```python
from build123d import *

# Parameters (mm, degrees)
SKETCH1_R                    = 9.5
BOSS_EXTRUDE1_DEPTH          = 10
CHAMFER1_SIZE                = 0.75
CIRPATTERN1_COUNT            = 12
CHAMFER1_OF_CIRPATTERN1_SIZE = 0.75
SKETCH2_R                    = 7
SKETCH2_R_2                  = 4.5
CUT_EXTRUDE1_DEPTH           = 2
FILLET1_R                    = 1
FILLET1_OF_MIRROR1_R         = 1
CUT_EXTRUDE2_REACH           = 12


with BuildPart() as part:
    # Sketch1 → Boss-Extrude1 (new body)
    with BuildSketch(Plane.XY):
        Circle(SKETCH1_R)
        with BuildLine():
            ThreePointArc((-2.07, 9.271736623), (0, 9.5), (2.07, 9.271736623))
            ThreePointArc((2.07, 9.271736623), (1.625653209, 11.72726856), (0.57, 13.988391616))
            ThreePointArc((0.57, 13.988391616), (0, 14), (-0.57, 13.988391616))
            ThreePointArc((-0.57, 13.988391616), (-1.625653209, 11.72726856), (-2.07, 9.271736623))
        make_face()
    boss_extrude1 = extrude(amount=BOSS_EXTRUDE1_DEPTH)

    # Chamfer1
    chamfer1_edges = [part.edges().sort_by_distance(p)[0] for p in [
        (0, 14, 10),
        (0, 14, 0),
    ]]
    chamfer(chamfer1_edges, length=CHAMFER1_SIZE)

    # CirPattern1: Boss-Extrude1 ×12 about axis
    cirpattern1_axis = Axis((0, 0, 0), (0, 0, 1))
    for i in range(1, CIRPATTERN1_COUNT):
        add(boss_extrude1.rotate(cirpattern1_axis, i * 360 / CIRPATTERN1_COUNT))

    # Chamfer1 of CirPattern1
    chamfer1_of_cirpattern1_edges = [part.edges().sort_by_distance(p)[0] for p in [
        (-7, 12.124355653, 10),
        (-7, 12.124355653, 0),
        (-12.124355653, 7, 10),
        (-12.124355653, 7, 0),
        (-14, 0, 10),
        (-14, 0, 0),
        (-12.124355653, -7, 10),
        (-12.124355653, -7, 0),
        (-7, -12.124355653, 10),
        (-7, -12.124355653, 0),
        (0, -14, 10),
        (0, -14, 0),
        (7, -12.124355653, 10),
        (7, -12.124355653, 0),
        (12.124355653, -7, 10),
        (12.124355653, -7, 0),
        (14, 0, 10),
        (14, 0, 0),
        (12.124355653, 7, 10),
        (12.124355653, 7, 0),
        (7, 12.124355653, 10),
        (7, 12.124355653, 0),
    ]]
    chamfer(chamfer1_of_cirpattern1_edges, length=CHAMFER1_OF_CIRPATTERN1_SIZE)

    # Sketch2 → Cut-Extrude1 (cut)
    with BuildSketch(Plane.XY.offset(10)):
        Circle(SKETCH2_R)
        Circle(SKETCH2_R_2, mode=Mode.SUBTRACT)
    cut_extrude1 = extrude(amount=-CUT_EXTRUDE1_DEPTH, mode=Mode.SUBTRACT)

    # Fillet1
    fillet1_edges = [part.edges().sort_by_distance(p)[0] for p in [
        (-7, 0, 8),
        (-4.5, 0, 8),
    ]]
    fillet(fillet1_edges, radius=FILLET1_R)

    # Mirror1: Cut-Extrude1 across plane
    add(cut_extrude1.mirror(Plane.XY.offset(5)), mode=Mode.SUBTRACT)

    # Fillet1 of Mirror1
    fillet1_of_mirror1_edges = [part.edges().sort_by_distance(p)[0] for p in [
        (-7, 0, 2),
        (-4.5, 0, 2),
    ]]
    fillet(fillet1_of_mirror1_edges, radius=FILLET1_OF_MIRROR1_R)

    # Sketch3 → Cut-Extrude2 (cut, up to next)
    with BuildSketch(Plane.XY.offset(10), mode=Mode.PRIVATE) as cut_extrude2_sk1:
        with BuildLine():
            Line((1.2489996, 1), (-1.2489996, 1))
            ThreePointArc((-1.2489996, 1), (-0.529905954, -1.509701851), (1.6, 0))
            ThreePointArc((1.6, 0), (1.509701851, 0.529905954), (1.2489996, 1))
        make_face()
    cut_extrude2_tool1 = extrude(cut_extrude2_sk1.sketch, amount=-CUT_EXTRUDE2_REACH, mode=Mode.PRIVATE) & part.part
    add(cut_extrude2_tool1.solids().sort_by_distance((0, -0.185603, 10))[0], mode=Mode.SUBTRACT)


solid = part.part
```
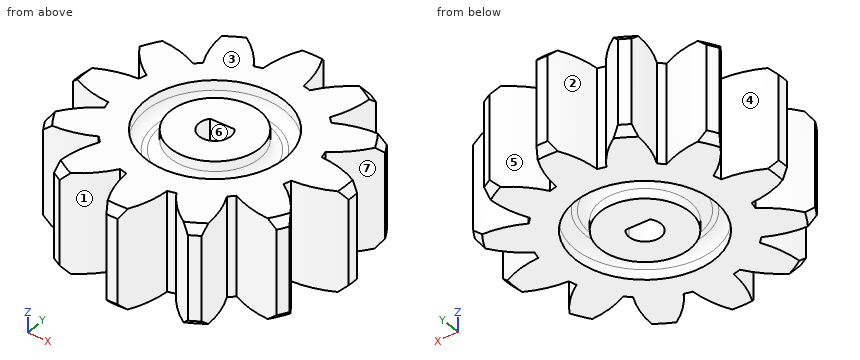
The model under review builds one solid part; all positions refer to its coordinate system, in mm. Face numbers are marked on the shaded views. A direction names the side the tool comes from. Give positions to 0.01 mm unless a question says otherwise; leave off trailing zeros. Loops run counter-clockwise (first coordinate to the right, second up) from the corner with the lowest first, then second, coordinate; pieces in that order, holes last. Notation, with made-up numbers: (77, 55) -> (130, 55) arc R34 cw to (130, 86) -> close; hole circle Ø6 at (-33, 3). An arc over 180 degrees is marked (long way). Use CSV: the item, a comma, the result in double quotes.
1. Machinability: for the marked faces 5, 6 and 7, which of the approach directions +Z, -Z, +X, -X, +Y, -Y give a long, thin tool a straight path to every point of the face, cutting with its end or side? Answer none if there is none.
Result:
face 5,"+Z, -Z, +Y"
face 6,"+Z, -Z"
face 7,"+Z, -Z, +X"
2. Consider section B-B, the plane y = 8. Write out the cut boundary in (x, z), then the cut area to 3 significant figures.
Result:
outline,"(-6.87, 0) -> (6.87, 0) -> (6.87, 10) -> (-6.87, 10) -> close"
area,"137 mm²"
3. The part is to be moulded in two halves that separate along Y. For the marked faces 1, 2, 3 and 4, say which applies: +Y half, -Y half, draft (parallel to the pull), parting line (faces both ways), or undercut.
Result:
face 1,"-Y half"
face 2,"+Y half"
face 3,"draft"
face 4,"undercut"
4. Consider section A-A, the plane z = 1.5. Count the separate pieces of the cut face and the enclosed holes in it, then the cut area to 3 significant figures.
Result:
separate pieces,"2"
enclosed holes,"2"
area,"363 mm²"
5. For P1, Ø6, axis at x = -4, z = 9, coming from the +Y side; P2, Ø1, axis at y = -8.5, z = 3, coming from the +X side; P3, Ø5, axis at y = -4.5, z = 2, coming from the +X side, all flat-tipped, find the tip position at first contact; note any pin that passes through.
Result:
P1,"stops at y = 13.24"
P2,"stops at x = 7.19"
P3,"stops at x = 12.4"
6. To check wall thickness, follow probe 1 along Y at (x, z) = (0, 5.75); probe 2 along X at (y, z) = (-1.25, 8.25); probe 3 along X at (y, z) = (-9.5, 1). State the ranges of each line that lie inside material, in increasing order. Write a range as from..to.
Result:
probe 1,"y = -14..-1.6, 1..14"
probe 2,"x = -12.72..-6.54, -4.67..-1, 1..4.67, 6.54..12.72"
probe 3,"x = -7.3..-3.14, -2.06..2.06, 3.14..7.3"
